Read the model definition and answer for the solid it produces. Units are mm, in the model's axes. A direction names the side the tool comes from. Coordinates: 2 decimals unless noted, no trailing zeros. Order: outer loops, then holes, each group sorted by start corner. A loop starts at its lowest first (then second) coordinate and runs counter-clockwise, first axis right, second up. Notation, with made-up numbers: (35, -40) - (39, -40) arc R19 ccw to (39, -20) - close; hole circle Ø3 at (13.5, 18). An arc over 180 degrees is marked (long way). Answer as a JSON object with one key per item and string values. Group by question number.
from build123d import *

# Parameters (mm, degrees)
SKETCH1_W                                        = 130
SKETCH1_H                                        = 110
BOSS_EXTRUDE1_DEPTH                              = 3
CBORE_FOR_M3_PAN_HEAD_MACHINE_SCREW1_D           = 3.4
CBORE_FOR_M3_PAN_HEAD_MACHINE_SCREW1_DEPTH       = 7
CBORE_FOR_M3_PAN_HEAD_MACHINE_SCREW1_CBORE_D     = 7
CBORE_FOR_M3_PAN_HEAD_MACHINE_SCREW1_CBORE_DEPTH = 2.4
CBORE_FOR_M3_PAN_HEAD_MACHINE_SCREW1_TIP         = 1.021463052
SKETCH10_W                                       = 25
SKETCH10_H                                       = 25
CUT_EXTRUDE1_DEPTH                               = 5
FILLET1_R                                        = 5


with BuildPart() as part:
    # Sketch1 → Boss-Extrude1 (new body)
    with BuildSketch(Plane(origin=(0, 0, 0), x_dir=(1, 0, 0), z_dir=(0, 1, 0))):
        with Locations((65, 55)):
            Rectangle(SKETCH1_W, SKETCH1_H)
    extrude(amount=BOSS_EXTRUDE1_DEPTH)

    # CBORE for M3 Pan Head Machine Screw1
    with Locations(Plane(origin=(0, 3, 0), x_dir=(1, 0, 0), z_dir=(0, 1, 0))):
        with Locations((5, 105), (125, 105), (125, 5), (5, 5)):
            CounterBoreHole(CBORE_FOR_M3_PAN_HEAD_MACHINE_SCREW1_D / 2, CBORE_FOR_M3_PAN_HEAD_MACHINE_SCREW1_CBORE_D / 2, CBORE_FOR_M3_PAN_HEAD_MACHINE_SCREW1_CBORE_DEPTH, depth=CBORE_FOR_M3_PAN_HEAD_MACHINE_SCREW1_DEPTH)
            with Locations((0, 0, -(CBORE_FOR_M3_PAN_HEAD_MACHINE_SCREW1_DEPTH + CBORE_FOR_M3_PAN_HEAD_MACHINE_SCREW1_TIP / 2))):  # 118° drill point
                Cone(0, CBORE_FOR_M3_PAN_HEAD_MACHINE_SCREW1_D / 2, CBORE_FOR_M3_PAN_HEAD_MACHINE_SCREW1_TIP, mode=Mode.SUBTRACT)

    # Sketch10 → Cut-Extrude1 (cut)
    with BuildSketch(Plane(origin=(0, 3, 0), x_dir=(1, 0, 0), z_dir=(0, 1, 0))):
        with Locations((82.5, 55)):
            Rectangle(SKETCH10_W, SKETCH10_H)
    extrude(amount=-CUT_EXTRUDE1_DEPTH, mode=Mode.SUBTRACT)

    # Fillet1
    fillet1_edges = [part.edges().sort_by_distance(p)[0] for p in [
        (0, 1.5, -110),
        (130, 1.5, -110),
        (130, 1.5, 0),
        (0, 1.5, 0),
    ]]
    fillet(fillet1_edges, radius=FILLET1_R)


solid = part.part
1. For faces 1 (the cylindrical face through (128, 2, -109)), 2 (the flat face through (82, 2, -42.5)), 3 (the cylindrical face through (128.233, 1.817, -103.659)), determine the directions among +Z, -Z, +X, -X, +Y, -Y from which every point of the face is accessible in a straight line to the end or side of a thin tool.
2. Given pin 1 (3.5 mm diameter, centred on x = 4, z = -6, fed in from +Y), flat-ended and moving along its own axis, determine where the tip first touches the part or whether it passes through.
3. Straight lines are drawn through the part: L1, parallel to Z at x = 125, y = 0.5; L2, parallel to X at y = 0.45, z = -105; L3, parallel to Z at x = 125, y = 1.3. For each, find the intervals that lie inside material, in ascending order.
4. A cutting plane is placed at A-A on y = 2. Write down the section's boundary in (x, z).
5. A cutting plane is placed at C-C on x = 80. Write down the section's boundary in (y, z).
6. For a pull along X with two mould halves and no side action, classify faces 4 (the cylindrical face through (8.233, 1.817, -3.659)), 5 (the cylindrical face through (1, 2, -2)), 6 (the flat face through (130, 1, -54)), 7 (the flat face through (64, 1, 0)) as pulls with the +X half, pulls with the -X half, needs draft (parallel to the pull), parting line crosses it, or undercut.
7. A cutting plane is placed at B-B on z = -51.5. Write down the section's boundary in (x, y).
Derived:
{
 "1": {"face 1": "-Z, +X, +Y, -Y", "face 2": "+Y, -Y", "face 3": "+Y"},
 "2": {"pin 1": "stops at y = 0.6"},
 "3": {"L1": "z = -110 to -106.7, -103.3 to -6.7, -3.3 to 0", "L2": "x = 0 to 3.3, 6.7 to 123.3, 126.7 to 130", "L3": "z = -110 to -108.5, -101.5 to -8.5, -1.5 to 0"},
 "4": {"outline": "(0, -105) arc R5 ccw to (5, -110) - (125, -110) arc R5 ccw to (130, -105) - (130, -5) arc R5 ccw to (125, 0) - (5, 0) arc R5 ccw to (0, -5) - close; hole circle Ø7 at (5, -105); hole circle Ø7 at (5, -5); hole (70, -67.5) - (95, -67.5) - (95, -42.5) - (70, -42.5) - close; hole circle Ø7 at (125, -105); hole circle Ø7 at (125, -5)"},
 "5": {"outline": "(0, -110) - (3, -110) - (3, -67.5) - (0, -67.5) - close; (0, -42.5) - (3, -42.5) - (3, 0) - (0, 0) - close"},
 "6": {"face 4": "undercut", "face 5": "pulls with the -X half", "face 6": "pulls with the +X half", "face 7": "needs draft"},
 "7": {"outline": "(0, 0) - (70, 0) - (70, 3) - (0, 3) - close; (95, 0) - (130, 0) - (130, 3) - (95, 3) - close"}
}
